Design review of the part built by this model. Coordinates are the model's own, in mm. A direction names the side the tool comes from. Coordinates: 2 decimals unless noted, no trailing zeros. Write each loop counter-clockwise with the first axis right and the second up, starting at its lowest first coordinate (ties: lowest second). Pieces come first, ordered by that corner, then holes. Notation, with made-up numbers: (13.5, 61) - (49.5, 61) arc R22 cw to (49.5, 87) - close; hole circle Ø4 at (40, -2.5). An arc over 180 degrees is marked (long way). Answer as CSV lines item,"result". Start each with the question number.
Q1. Clearance check with flat-ended pins moving along their axes: pin 1 (5 mm diameter, centred on x = -16.51, z = 16.51, fed in from +Y); pin 2 (2 mm diameter, centred on x = 21.59, z = 21.59, fed in from +Y). State where each tip first meets the part, or that it passes through.
Q2. We need section B-B (x = -16.51). Write out the cut boundary in (y, z).
Q3. Mouldability with a two-part tool opening along X and no side actions: class faces 3 (the face through (0, 13, -25.4)), 4 (the face through (-25.4, 13, 0)), 5 (the face through (18, 17.475, -15)) as pulls with the +X half, pulls with the -X half, needs draft (parallel to the pull), parting line crosses it, or undercut.
Q4. We need section A-A (z = 16.51). Write out the cut boundary in (x, y).
Q5. For line 1 along X through (y, z) = (21, 16.51); line 2 along Z through (x, y) = (16.51, 9), list the stretches that pass through material, from the lowest coordinate up. Write a range as [from, to].
Q6. We need section C-C (y = 19). State how many separate pieces and enclosed holes the cut face has, plus the area to 3 significant figures.
Q7. Machinability: for faces 1 (the face through (16.864, 8.615, 18.103)), 2 (the face through (-18.715, 21.493, 18.201)), which of the approach directions +Z, -Z, +X, -X, +Y, -Y give a long, thin tool a straight path to every point of the face, cutting with its end or side? Answer none if there is none.
from build123d import *

# Parameters (mm, degrees)
SKETCH1_W                                      = 50.8
SKETCH1_H                                      = 50.8
BOSS_EXTRUDE1_DEPTH                            = 25.4
F_4_40_TAPPED_HOLE1_D                          = 2.2606
F_4_40_TAPPED_HOLE1_DEPTH                      = 20.2946
F_4_40_TAPPED_HOLE1_TIP                        = 0.679152758
CBORE_FOR_4_SOCKET_HEAD_CAP_SCREW1_D           = 3.2639
CBORE_FOR_4_SOCKET_HEAD_CAP_SCREW1_CBORE_D     = 5.55752
CBORE_FOR_4_SOCKET_HEAD_CAP_SCREW1_CBORE_DEPTH = 7.9248


with BuildPart() as part:
    # Sketch1 → Boss-Extrude1 (new body)
    with BuildSketch(Plane(origin=(0, 0, 0), x_dir=(1, 0, 0), z_dir=(0, 1, 0))):
        Rectangle(SKETCH1_W, SKETCH1_H)
    extrude(amount=BOSS_EXTRUDE1_DEPTH)

    # #4-40 Tapped Hole1
    with Locations(Plane(origin=(0, 25.4, 0), x_dir=(1, 0, 0), z_dir=(0, 1, 0))):
        with Locations((-21.59, 21.59), (21.59, 21.59), (21.59, -21.59), (-21.59, -21.59)):
            Hole(F_4_40_TAPPED_HOLE1_D / 2, depth=F_4_40_TAPPED_HOLE1_DEPTH)
            with Locations((0, 0, -(F_4_40_TAPPED_HOLE1_DEPTH + F_4_40_TAPPED_HOLE1_TIP / 2))):  # 118° drill point
                Cone(0, F_4_40_TAPPED_HOLE1_D / 2, F_4_40_TAPPED_HOLE1_TIP, mode=Mode.SUBTRACT)

    # CBORE for #4 Socket Head Cap Screw1 (through all)
    with Locations(Plane(origin=(0, 25.4, 0), x_dir=(1, 0, 0), z_dir=(0, 1, 0))):
        with Locations((-16.51, 16.51), (16.51, 16.51), (16.51, -16.51), (-16.51, -16.51)):
            CounterBoreHole(CBORE_FOR_4_SOCKET_HEAD_CAP_SCREW1_D / 2, CBORE_FOR_4_SOCKET_HEAD_CAP_SCREW1_CBORE_D / 2, CBORE_FOR_4_SOCKET_HEAD_CAP_SCREW1_CBORE_DEPTH)


solid = part.part
Results list:
1,pin 1,"stops at y = 17.48"
1,pin 2,"stops at y = 5.03"
2,outline,"(0, -25.4) - (25.4, -25.4) - (25.4, -19.29) - (17.48, -19.29) - (17.48, -18.14) - (0, -18.14) - close; (0, -14.88) - (17.48, -14.88) - (17.48, -13.73) - (25.4, -13.73) - (25.4, 13.73) - (17.48, 13.73) - (17.48, 14.88) - (0, 14.88) - close; (0, 18.14) - (17.48, 18.14) - (17.48, 19.29) - (25.4, 19.29) - (25.4, 25.4) - (0, 25.4) - close"
3,face 3,"needs draft"
3,face 4,"pulls with the -X half"
3,face 5,"undercut"
4,outline,"(-25.4, 0) - (-18.14, 0) - (-18.14, 17.48) - (-19.29, 17.48) - (-19.29, 25.4) - (-25.4, 25.4) - close; (-14.88, 0) - (14.88, 0) - (14.88, 17.48) - (13.73, 17.48) - (13.73, 25.4) - (-13.73, 25.4) - (-13.73, 17.48) - (-14.88, 17.48) - close; (18.14, 0) - (25.4, 0) - (25.4, 25.4) - (19.29, 25.4) - (19.29, 17.48) - (18.14, 17.48) - close"
5,line 1,"x = [-25.4, -19.29], [-13.73, 13.73], [19.29, 25.4]"
5,line 2,"z = [-25.4, -18.14], [-14.88, 14.88], [18.14, 25.4]"
6,separate pieces,"1"
6,enclosed holes,"8"
6,area,"2,470 mm2"
7,face 1,"+Y, -Y"
7,face 2,"+Y"
